Design review of the part built by this model. Coordinates are the model's own, in mm. A direction names the side the tool comes from. Round coordinates to 2 decimals unless told otherwise and drop trailing zeros. Order: outer loops, then holes, each group sorted by start corner. A loop starts at its lowest first (then second) coordinate and runs counter-clockwise, first axis right, second up. Notation, with made-up numbers: (14, 66.25) - (51, 66.25) arc R21 cw to (51, 98.25) - close; hole circle Ø4 at (32.25, 79). An arc over 180 degrees is marked (long way). Answer as a JSON object with one key per item and string values. Group by question number.
from build123d import *

# Parameters (mm, degrees)
SKETCH1_R           = 11
BOSS_EXTRUDE1_DEPTH = 27.94
SKETCH2_R           = 10.4267
CUT_EXTRUDE1_DEPTH  = 1.1684


with BuildPart() as part:
    # Sketch1 → Boss-Extrude1 (new body)
    with BuildSketch(Plane(origin=(0, 0, 0), x_dir=(1, 0, 0), z_dir=(0, 1, 0))):
        Circle(SKETCH1_R)
    extrude(amount=BOSS_EXTRUDE1_DEPTH)

    # Sketch2 → Cut-Extrude1 (cut)
    with BuildSketch(Plane(origin=(0, 12.954, 0), x_dir=(1, 0, 0), z_dir=(0, 1, 0))):
        with BuildLine():
            Line((-17.239436612, 14.563425366), (-16.28375247, -14.840830381))
            Line((-16.28375247, -14.840830381), (21.406068048, -16.295664576))
            Line((21.406068048, -16.295664576), (22.094276354, 14.197317514))
            Line((22.094276354, 14.197317514), (19.887741586, 14.563425366))
            ThreePointArc((19.887741586, 14.563425366), (1.324152487, 14.86501853), (-17.239436612, 14.563425366))
        make_face()
        Circle(SKETCH2_R, mode=Mode.SUBTRACT)
    extrude(amount=-CUT_EXTRUDE1_DEPTH, mode=Mode.SUBTRACT)


solid = part.part
1. Clearance check with flat-ended pins moving along their axes: P1, Ø1.5, axis at y = 11, z = -8, coming from the -X side; P2, Ø6, axis at x = -3.5, y = 24, coming from the -Z side; P3, Ø8, axis at x = -4.5, y = 4, coming from the +Z side. State where each tip first meets the part, or that it passes through.
2. Tool access review of faces 4 (the cylindrical face through (-2.38, 5.81, 10.74)), 5 (the flat face through (-7, 11.786, 8)): name each direction out of +Z, -Z, +X, -X, +Y, -Y from which nothing blocks a thin tool from reaching the whole face with its end or side.
3. To check wall thickness, follow line 1 (Y direction, x = 6.75, z = -8.5); line 2 (Z direction, x = -3.5, y = 14.5); line 3 (X direction, y = 13.25, z = 8.5). State the ranges of each line that lie inside material, in increasing order. Write a range as from..to.
4. Take a section at A-A, the plane z = 9.5. Give the boundary of the cut face in (x, y).
5. Mouldability with a two-part tool opening along Y and no side actions: class faces 1 (the flat face through (-7, 12.954, 8)), 2 (the flat face through (0, 0, 0)), 3 (the cylindrical face through (-2.38, 20.34, 10.74)) as pulls with the +Y half, pulls with the -Y half, needs draft (parallel to the pull), parting line crosses it, or undercut.
6. Take a section at B-B, the plane x = -6.25. Give the boundary of the cut face in (y, z).
7. Take a section at C-C, the plane y = 10.75. Give the boundary of the cut face in (x, z).
Response values:
{
 "1": {"P1": "x = -8.27", "P2": "z = -10.99", "P3": "z = 10.99"},
 "2": {"face 4": "+Y, -Y", "face 5": "none"},
 "3": {"line 1": "0..11.79, 12.95..27.94", "line 2": "-10.43..10.43", "line 3": "-6.98..6.98"},
 "4": {"outline": "(-5.55, 0) - (5.55, 0) - (5.55, 11.79) - (4.3, 11.79) - (4.3, 12.95) - (5.55, 12.95) - (5.55, 27.94) - (-5.55, 27.94) - (-5.55, 12.95) - (-4.3, 12.95) - (-4.3, 11.79) - (-5.55, 11.79) - close"},
 "5": {"face 1": "undercut", "face 2": "pulls with the -Y half", "face 3": "needs draft"},
 "6": {"outline": "(0, -9.05) - (11.79, -9.05) - (11.79, -8.35) - (12.95, -8.35) - (12.95, -9.05) - (27.94, -9.05) - (27.94, 9.05) - (12.95, 9.05) - (12.95, 8.35) - (11.79, 8.35) - (11.79, 9.05) - (0, 9.05) - close"},
 "7": {"outline": "circle Ø22 at (0, 0)"}
}
